from build123d import *

# Parameters (mm, degrees)
F0_W      = 50
F0_H      = 90
F1_DEPTH  = 2
F2_R      = 28
F3_DEPTH  = 1.5
F4_R      = 28
F4_R_2    = 27
F5_DEPTH  = 1
F6_W      = 3
F6_H      = 70
F7_DEPTH  = 3
F8_DEPTH  = 3
F10_DEPTH = 25
F11_W     = 8
F11_H     = 6
F12_DEPTH = 25
F13_R     = 1
F14_R     = 1
F15_R     = 5
F18_SIZE  = 0.25
F19_R     = 28
F19_R_2   = 27.25
F19_R_3   = 26
F20_DEPTH = 0.5
F21_SIZE  = 0.24999
F22_R     = 28
F22_R_2   = 26.24999
F22_R_3   = 26
F23_DEPTH = 0.5
F24_SIZE  = 0.2499
F25_R     = 28
F25_R_2   = 26.2499
F25_R_3   = 26
F26_DEPTH = 0.5
F27_SIZE  = 0.249


# Not quite as in the source:
# - a fillet or chamfer is up to 0.001 mm smaller than in the source, because OpenCascade refuses the exact size


with BuildPart() as f1:
    # F0 (on Top) → F1 (new body)
    with BuildSketch(Plane.XY):
        Rectangle(F0_W, F0_H)
    extrude(amount=F1_DEPTH)

    # F2 (on face) → F3 (join)
    with BuildSketch(Plane.XY.offset(2)):
        Circle(F2_R)
    extrude(amount=F3_DEPTH)

    # F4 (on face) → F5 (join)
    with BuildSketch(Plane.XY.offset(3.5)):
        Circle(F4_R)
        Circle(F4_R_2, mode=Mode.SUBTRACT)
    extrude(amount=F5_DEPTH)

    # F6 (on face) → F7 (join)
    with BuildSketch(Plane(origin=(0, 0, 0), x_dir=(1, 0, 0), z_dir=(0, 0, -1))):
        with Locations((-23.5, 0)):
            Rectangle(F6_W, F6_H)
        with Locations((23.5, 0)):
            Rectangle(F6_W, F6_H)
    extrude(amount=F7_DEPTH)

    # F8 (cut, through all): faces of the model
    f8_faces = [f1.faces().sort_by_distance(p)[0] for p in [
        (-23.5, 0, -3),
        (23.5, 0, -3),
        (-23.5, 0, -3),
        (23.5, 0, -3),
    ]]
    extrude(f8_faces, amount=-F8_DEPTH, mode=Mode.SUBTRACT)

    # F9 (on face) → F10 (cut)
    with BuildSketch(Plane.XY.offset(3.5)):
        with BuildLine():
            Line((-5.6568542495, 0), (-14.8752109279, 9.2183566784))
            ThreePointArc((-14.8752109279, 9.2183566784), (-17.5, 0), (-14.8752109279, -9.2183566784))
            Line((-14.8752109279, -9.2183566784), (-5.6568542495, 0))
        make_face()
        with BuildLine():
            ThreePointArc((-9.2183566784, -14.8752109279), (0, -17.5), (9.2183566784, -14.8752109279))
            Line((9.2183566784, -14.8752109279), (0, -5.6568542495))
            Line((0, -5.6568542495), (-9.2183566784, -14.8752109279))
        make_face()
        with BuildLine():
            ThreePointArc((14.8752109279, -9.2183566784), (16.831015882, -4.7923798244), (17.5, 0))
            ThreePointArc((17.5, 0), (16.831015882, 4.7923798244), (14.8752109279, 9.2183566784))
            Line((14.8752109279, 9.2183566784), (5.6568542495, 0))
            Line((5.6568542495, 0), (14.8752109279, -9.2183566784))
        make_face()
        with BuildLine():
            Line((0, 5.6568542495), (9.2183566784, 14.8752109279))
            ThreePointArc((9.2183566784, 14.8752109279), (0, 17.5), (-9.2183566784, 14.8752109279))
            Line((-9.2183566784, 14.8752109279), (0, 5.6568542495))
        make_face()
    extrude(amount=-F10_DEPTH, mode=Mode.SUBTRACT)

    # F11 (on face) → F12 (cut)
    with BuildSketch(Plane(origin=(0, 0, 0), x_dir=(1, 0, 0), z_dir=(0, 0, -1))):
        with Locations((0, -42)):
            Rectangle(F11_W, F11_H)
        with BuildLine():
            Line((-4, -39), (4, -39))
            Line((4, -39), (19, -39))
            ThreePointArc((19, -39), (19.7071067812, -38.7071067812), (20, -38))
            Line((20, -38), (20, -34))
            ThreePointArc((20, -34), (19.7071067812, -33.2928932188), (19, -33))
            Line((19, -33), (-19, -33))
            ThreePointArc((-19, -33), (-19.7071067812, -33.2928932188), (-20, -34))
            Line((-20, -34), (-20, -38))
            ThreePointArc((-20, -38), (-19.7071067812, -38.7071067812), (-19, -39))
            Line((-19, -39), (-4, -39))
        make_face()
        with Locations((0, 42)):
            Rectangle(F11_W, F11_H)
        with BuildLine():
            ThreePointArc((20, 38), (19.7071067812, 38.7071067812), (19, 39))
            Line((19, 39), (4, 39))
            Line((4, 39), (-4, 39))
            Line((-4, 39), (-19, 39))
            ThreePointArc((-19, 39), (-19.7071067812, 38.7071067812), (-20, 38))
            Line((-20, 38), (-20, 34))
            ThreePointArc((-20, 34), (-19.7071067812, 33.2928932188), (-19, 33))
            Line((-19, 33), (19, 33))
            ThreePointArc((19, 33), (19.7071067812, 33.2928932188), (20, 34))
            Line((20, 34), (20, 38))
        make_face()
    extrude(amount=-F12_DEPTH, mode=Mode.SUBTRACT)

    # F13
    f13_edges = [f1.edges().sort_by_distance(p)[0] for p in [
        (-4, -45, 1),
        (-4, -39, 1),
        (4, -45, 1),
        (4, -39, 1),
    ]]
    fillet(f13_edges, radius=F13_R)

    # F14
    f14_edges = [f1.edges().sort_by_distance(p)[0] for p in [
        (4, 45, 1),
        (4, 39, 1),
        (-4, 45, 1),
        (-4, 39, 1),
    ]]
    fillet(f14_edges, radius=F14_R)

    # F15
    f15_edges = [f1.edges().sort_by_distance(p)[0] for p in [
        (25, -45, 1),
        (25, 45, 1),
        (-25, 45, 1),
        (-25, -45, 1),
    ]]
    fillet(f15_edges, radius=F15_R)


with BuildPart() as f16_1:
    # F16: copy of F1
    add(f1.part.moved(Location((72.1, 0, 0))))


with BuildPart() as f1_1:
    add(f1.part)

    # F18
    f18_edges = [f1_1.edges().sort_by_distance(p)[0] for p in [
        (-27, 0, 4.5),
    ]]
    chamfer(f18_edges, length=F18_SIZE)

    # F19 (on face) → F20 (join)
    with BuildSketch(Plane.XY.offset(4.5)):
        Circle(F19_R)
        Circle(F19_R_2, mode=Mode.SUBTRACT)
        Circle(F19_R_2)
        Circle(F19_R_3, mode=Mode.SUBTRACT)
    extrude(amount=F20_DEPTH)

    # F21 (size 0.25 in the source; OpenCascade refuses exactly that, so slightly less here)
    f21_edges = [f1_1.edges().sort_by_distance(p)[0] for p in [
        (-26, 0, 4.5),
        (-26, 0, 5),
    ]]
    chamfer(f21_edges, length=F21_SIZE)

    # F22 (on face) → F23 (join)
    with BuildSketch(Plane.XY.offset(5)):
        Circle(F22_R)
        Circle(F22_R_2, mode=Mode.SUBTRACT)
        Circle(F22_R_2)
        Circle(F22_R_3, mode=Mode.SUBTRACT)
    extrude(amount=F23_DEPTH)

    # F24 (size 0.25 in the source; OpenCascade refuses exactly that, so slightly less here)
    f24_edges = [f1_1.edges().sort_by_distance(p)[0] for p in [
        (-26, 0, 5),
        (-26, 0, 5.5),
    ]]
    chamfer(f24_edges, length=F24_SIZE)

    # F25 (on face) → F26 (join)
    with BuildSketch(Plane.XY.offset(5.5)):
        Circle(F25_R)
        Circle(F25_R_2, mode=Mode.SUBTRACT)
        Circle(F25_R_2)
        Circle(F25_R_3, mode=Mode.SUBTRACT)
    extrude(amount=F26_DEPTH)

    # F27 (size 0.25 in the source; OpenCascade refuses exactly that, so slightly less here)
    f27_edges = [f1_1.edges().sort_by_distance(p)[0] for p in [
        (-26, 0, 6),
        (-26, 0, 5.5),
    ]]
    chamfer(f27_edges, length=F27_SIZE)


solid = f1_1.part
CAD build for the part. Positions are in the model's coordinates, mm. A direction names the side the tool comes from. Coordinates: 2 decimals unless noted, no trailing zeros. Order: outer loops, then holes, each group sorted by start corner. A loop starts at its lowest first (then second) coordinate and runs counter-clockwise, first axis right, second up.
Item 1: Pin check, flat tips, straight feed: pin 1 Ø0.6 at (y, z) = (-19.5, 1) entering from -X; pin 2 Ø1 at (y, z) = (-42.5, 1.5) entering from +X; pin 3 Ø1.5 at (x, y) = (26, -6) entering from -Z. Stop position of each tip, or through.
Check sheet entries:
pin 1: stops at x = -25
pin 2: stops at x = 24.58
pin 3: stops at z = 2
Item 2: Band-saw the part on B-B on z = 1. Give the number of separate pieces and of enclosed holes in the cut face, plus the area to 3 significant figures.
Check sheet entries:
separate pieces: 1
enclosed holes: 4
area: 3,430 mm2
Item 3: Band-saw the part on A-A on y = 36. List the corners of the cut face in (x, z).
Check sheet entries:
outline: (-25, 0) - (-20, 0) - (-20, 2) - (-25, 2) - close; (20, 0) - (25, 0) - (25, 2) - (20, 2) - close
Item 4: 3-axis set-ups, long thin cutter, end or side, ignore diameter. For faces 1 (the face through (-26, 0, 2)), 2 (the face through (4, -42, 1)), 3 (the face through (26, 0, 2)), 4 (the face through (-4.545, -10.202, 1.774)): which of +Z, -Z, +X, -X, +Y, -Y reach the whole face in a straight line?
Check sheet entries:
face 1: -Z, -X, +Y, -Y
face 2: +Z, -Z, -Y
face 3: -Z, +X, +Y, -Y
face 4: +Z, -Z
Item 5: Two-plate mould, pull along Y, no slides. Class faces 5 (the face through (4, 42, 1)), 6 (the face through (25.865, -10.724, 3.972)), 7 (the face through (12, 39, 1)): +Y half, -Y half, draft (parallel to the pull), parting line (faces both ways), or undercut.
Check sheet entries:
face 5: draft
face 6: parting line
face 7: undercut
Item 6: Drill centre lines: L1, parallel to Y at x = 0, z = 4.75; L2, parallel to Y at x = -16, z = 1.95; L3, parallel to Y at x = 8, z = 1.55. Where is each one in solid material? Low to high.
Check sheet entries:
L1: y = -28 to -26, 26 to 28
L2: y = -45 to -39, -33 to -7.09, 7.09 to 33, 39 to 45
L3: y = -45 to -39, -33 to -15.56, -13.66 to -2.34, 2.34 to 13.66, 15.56 to 33, 39 to 45
